Source: three-view drawing plus pictorial views. Frame: mm from the lowest corner of the part. A direction names the side the tool comes from. Coordinates: 2 decimals unless noted, no trailing zeros. Loops run counter-clockwise (first coordinate to the right, second up) from the corner with the lowest first, then second, coordinate; pieces in that order, holes last.
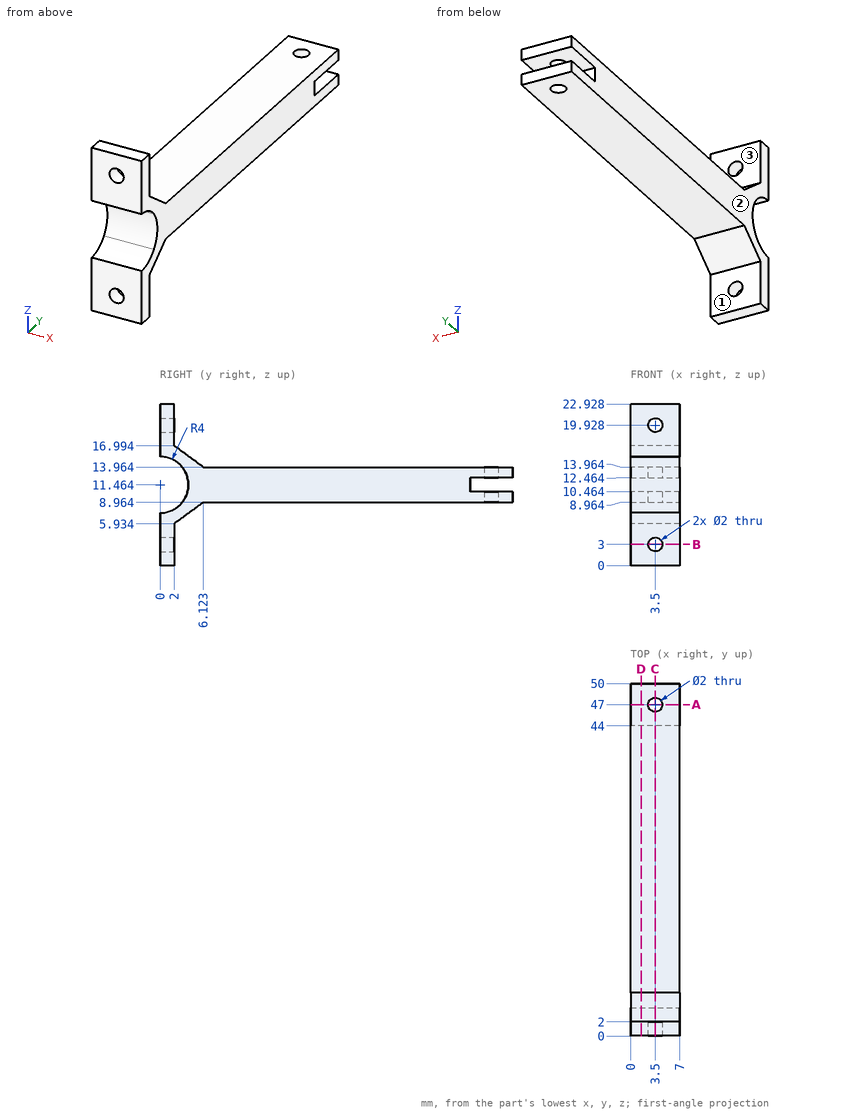
Q1. Section D-D, the plane x = 1.5. Return the cut outline in (y, z) (1 decimal).
Q2. Section B-B, the plane z = 3. Return the cut outline in (x, y), plus the area to 3 significant figures.
Q3. Line query: line 1 along Z through (x, y) = (6, 44.5) (1 decimal); line 2 along Z through (x, y) = (3.5, 0.9); line 3 along Y through (x, z) = (6.25, 3.5). Output: solid intervals per line, ascending.
Q4. Contact query for flat-ended pins moving along their axis: pin 1 Ø4 at (x, y) = (6.5, 37) entering from +Z; pin 2 Ø4 at (x, y) = (6, 37) entering from -Z; pin 3 Ø1.8 at (x, z) = (2.5, 2) entering from +Y. Output: stop coordinate, or through.
Q5. Section A-A, the plane y = 47. Return the cut outline in (x, z) (1 decimal), plus the area to 3 significant figures.
Q6. Access query for the marked faces 1, 2 and 3. Directions: +Z, -Z, +X, -X, +Y, -Y. A direction counts if a zero-diameter tool reaches every point of the face in a straight line with its end or side. Return the directions, or none.
Q7. Section C-C, the plane x = 3.5. Count the separate pieces of the cut face and the enclosed holes in it, plus the area to 3 significant figures.
Derived:
1. outline: (0, 0) - (2, 0) - (2, 5.9) - (6.1, 9) - (50, 9) - (50, 10.5) - (44, 10.5) - (44, 12.5) - (50, 12.5) - (50, 14) - (6.1, 14) - (2, 17) - (2, 22.9) - (0, 22.9) - (0, 15.5) arc R4 cw to (3.1, 14) arc R4 cw to (3.1, 9) arc R4 cw to (0, 7.5) - close
2. outline: (0, 0) - (2.5, 0) - (2.5, 2) - (0, 2) - close; (4.5, 0) - (7, 0) - (7, 2) - (4.5, 2) - close
2. area: 10.0 mm2
3. line 1: z = 9 to 10.5, 12.5 to 14
3. line 2: z = 0 to 2, 4 to 7.57, 15.36 to 18.93, 20.93 to 22.93
3. line 3: y = 0 to 2
4. pin 1: stops at z = 13.96
4. pin 2: stops at z = 8.96
4. pin 3: stops at y = 2
5. outline: (0, 9) - (2.5, 9) - (2.5, 10.5) - (0, 10.5) - close; (0, 12.5) - (2.5, 12.5) - (2.5, 14) - (0, 14) - close; (4.5, 9) - (7, 9) - (7, 10.5) - (4.5, 10.5) - close; (4.5, 12.5) - (7, 12.5) - (7, 14) - (4.5, 14) - close
5. area: 15.0 mm2
6. face 1: -Z, +X, -X, +Y
6. face 2: +Z, -Z, -X, +Y, -Y
6. face 3: +Z, +X, -X, +Y
7. separate pieces: 5
7. enclosed holes: 0
7. area: 247 mm2
